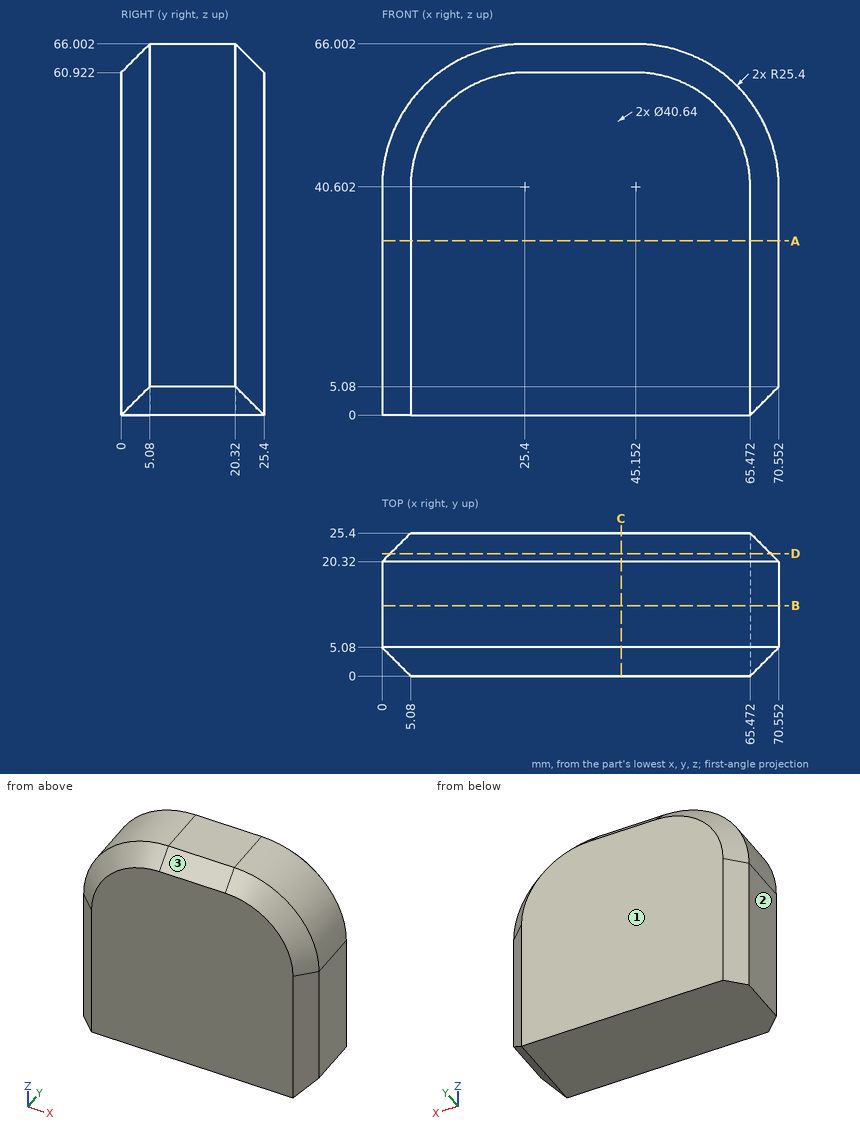
Design review of the part shown in the three views and the two pictorial views. Dimensions are in mm from the part's minimum x, y and z. Coordinates: 2 decimals unless noted, no trailing zeros. Order: outer loops, then holes, each group sorted by start corner. A loop starts at its lowest first (then second) coordinate and runs counter-clockwise, first axis right, second up.
Item 1: The part is to be moulded in two halves that separate along Y. For the marked faces 1, 2 and 3, say which applies: pulls with the +Y half, pulls with the -Y half, needs draft (parallel to the pull), parting line crosses it, or undercut.
Item 2: Take a section at C-C, the plane x = 42.5. Write out the cut boundary in (y, z), then the cut area to 3 significant figures.
Item 3: For line 1 (Z direction, x = 56, y = 9); line 2 (Z direction, x = 57, y = 6.25); line 3 (X direction, y = 4.75, z = 51) (1 decimal), list the stretches that pass through material, from the lowest coordinate up.
Item 4: For pin 1 Ø2 at (y, z) = (3.5, 19) entering from +X; pin 2 Ø8 at (x, y) = (18.5, 22) entering from +Z; pin 3 Ø5 at (x, y) = (15.5, 11) entering from +Z, all flat-tipped, find the tip position at first contact; note any pin that passes through.
Item 5: Take a section at B-B, the plane y = 12.5. Write out the cut boundary in (x, z), then the cut area to 3 significant figures.
Item 6: Take a section at A-A, the plane z = 31. Write out the cut boundary in (x, y).
Item 7: Take a section at D-D, the plane y = 21.75. Write out the cut boundary in (x, z).
The answers:
1. face 1: pulls with the +Y half
1. face 2: needs draft
1. face 3: pulls with the -Y half
2. outline: (0, 0) - (25.4, 0) - (25.4, 60.92) - (20.32, 66) - (5.08, 66) - (0, 60.92) - close
2. area: 1,650 mm2
3. line 1: z = 0 to 63.57
3. line 2: z = 0 to 63.07
3. line 3: x = 2.6 to 68
4. pin 1: stops at x = 69.97
4. pin 2: stops at z = 65.79
4. pin 3: stops at z = 64.9
5. outline: (0, 0) - (65.47, 0) - (70.55, 5.08) - (70.55, 40.6) arc R25.4 ccw to (45.15, 66) - (25.4, 66) arc R25.4 ccw to (0, 40.6) - close
5. area: 4,370 mm2
6. outline: (0, 5.08) - (5.08, 0) - (65.47, 0) - (70.55, 5.08) - (70.55, 20.32) - (65.47, 25.4) - (5.08, 25.4) - (0, 20.32) - close
7. outline: (1.43, 0) - (65.47, 0) - (69.12, 3.65) - (69.12, 40.6) arc R23.97 ccw to (45.15, 64.57) - (25.4, 64.57) arc R23.97 ccw to (1.43, 40.6) - close
